from build123d import *

# Parameters (mm, degrees)
EXTRUDE_1_DEPTH     = 3
SKETCH_2_R          = 2.025
CUT_EXTRUDE_1_DEPTH = 3
SKETCH_3_W          = 30
SKETCH_3_H          = 18
SKETCH_3_W_2        = 22
SKETCH_3_H_2        = 15
CUT_EXTRUDE_2_DEPTH = 3
FILLET_1_R          = 2
FILLET_2_R          = 3


with BuildPart() as part:
    # 草图1 → 凸台-拉伸1 (new body)
    with BuildSketch(Plane.XY):
        Polygon((-40, 0), (40, 0), (40, -30), (20, -70), (-20, -70), (-40, -30), align=None)
    extrude(amount=EXTRUDE_1_DEPTH)

    # 草图2 → 切除-拉伸1 (cut)
    with BuildSketch(Plane.XY.offset(3)):
        with Locations((-25, -15)):
            Circle(SKETCH_2_R)
        with Locations((25, -15)):
            Circle(SKETCH_2_R)
        with Locations((0, -35)):
            Circle(SKETCH_2_R)
        with Locations((12.5, -60)):
            Circle(SKETCH_2_R)
        with Locations((-12.5, -60)):
            Circle(SKETCH_2_R)
    extrude(amount=-CUT_EXTRUDE_1_DEPTH, mode=Mode.SUBTRACT)

    # 草图3 → 切除-拉伸2 (cut)
    with BuildSketch(Plane.XY.offset(3)):
        Polygon((-34.409830056, -30), (-20, -30), (-20, -58.819660113), align=None)
        with Locations((0, -15)):
            Rectangle(SKETCH_3_W, SKETCH_3_H)
        with Locations((0, -47.5)):
            Rectangle(SKETCH_3_W_2, SKETCH_3_H_2)
        Polygon((20, -30), (20, -58.819660113), (34.409830056, -30), align=None)
    extrude(amount=-CUT_EXTRUDE_2_DEPTH, mode=Mode.SUBTRACT)

    # 圆角1
    fillet_1_edges = [part.edges().sort_by_distance(p)[0] for p in [
        (15, -24, 1.5),
        (-15, -24, 1.5),
        (-15, -6, 1.5),
        (15, -6, 1.5),
        (-20, -58.819660113, 1.5),
        (-34.409830056, -30, 1.5),
        (-20, -30, 1.5),
        (11, -55, 1.5),
        (-11, -55, 1.5),
        (-11, -40, 1.5),
        (11, -40, 1.5),
        (34.409830056, -30, 1.5),
        (20, -58.819660113, 1.5),
        (20, -30, 1.5),
    ]]
    fillet(fillet_1_edges, radius=FILLET_1_R)

    # 圆角2
    fillet_2_edges = [part.edges().sort_by_distance(p)[0] for p in [
        (-40, 0, 1.5),
        (40, 0, 1.5),
        (40, -30, 1.5),
        (20, -70, 1.5),
        (-20, -70, 1.5),
        (-40, -30, 1.5),
    ]]
    fillet(fillet_2_edges, radius=FILLET_2_R)


solid = part.part
Can you work these out from the model? Positions are in its coordinate system, mm. A direction names the side the tool comes from. Give positions to 0.01 mm unless a question says otherwise; leave off trailing zeros. Order: outer loops, then holes, each group sorted by start corner. A loop starts at its lowest first (then second) coordinate and runs counter-clockwise, first axis right, second up. Notation, with made-up numbers: M 13,11 L 65,11 A20 cw 65,22 Z; hole C 35.5,25.25 d6. An arc over 180 degrees is marked long. Use one line per item in the form item = value.
Item 1: For faces 1 (the flat face through (-30, -50, 1)), 2 (the cylindrical face through (10.4, -40.57, 1.48)), which set-ups out of +Z, -Z, +X, -X, +Y, -Y let a thin tool reach every point of the face, with its end or its side?
Values follow:
face_1 = +Z, -Z, -X, -Y
face_2 = +Z, -Z
Item 2: If we section it at C-C, the plane z = 1.35: Count the separate pieces of the cut face and the enclosed holes in it, and give its area (3 significant figures).
Values follow:
separate_pieces = 1
enclosed_holes = 9
area = 3,480 mm^2
Item 3: If we section it at B-B, the plane x = -8: Write out the boundary of the cut face in (y, z).
Values follow:
outline = M -70,0 L -55,0 L -55,3 L -70,3 Z; M -40,0 L -24,0 L -24,3 L -40,3 Z; M -6,0 L 0,0 L 0,3 L -6,3 Z
Item 4: Will these pins go through, and if not, where does the flat tip stop? pin 1 Ø5.5 at (x, y) = (25, -15) entering from -Z; pin 2 Ø1.5 at (y, z) = (-37, 2) entering from -X (3 decimals); pin 3 Ø1.5 at (y, z) = (-49, 1) entering from -X (3 decimals).
Values follow:
pin_1 = 0
pin_2 = -36.875
pin_3 = -30.875
Item 5: If we section it at A-A, the plane y = -15: Write out the boundary of the cut face in (x, z) (3 decimals), and give its area (3 significant figures).
Values follow:
outline = M -40,0 L -27.025,0 L -27.025,3 L -40,3 Z; M -22.975,0 L -15,0 L -15,3 L -22.975,3 Z; M 15,0 L 22.975,0 L 22.975,3 L 15,3 Z; M 27.025,0 L 40,0 L 40,3 L 27.025,3 Z
area = 126 mm^2
Item 6: If we section it at D-D, the plane x = 28: Write out the boundary of the cut face in (y, z).
Values follow:
outline = M -54,0 L -42.82,0 L -42.82,3 L -54,3 Z; M -30,0 L 0,0 L 0,3 L -30,3 Z
Item 7: If I drill on line 1 along Y through (x, z) = (12.5, 1.3) (3 decimals); line 2 along Y through (x, z) = (-26, 1.75); line 3 along Y through (x, z) = (0.5, 1.75), over which ranges is the centre line in solid material (lowest first)? Write a range as [from, to].
Values follow:
line_1 = [-70, -62.025], [-57.975, -24], [-6, 0]
line_2 = [-58, -46.82], [-30, -16.76], [-13.24, 0]
line_3 = [-70, -55], [-40, -36.96], [-33.04, -24], [-6, 0]
